Source: CAD feature listing. Evaluate the final solid. Frame: model axes, mm. A direction names the side the tool comes from. Give positions to 0.01 mm unless a question says otherwise; leave off trailing zeros. Loops run counter-clockwise (first coordinate to the right, second up) from the corner with the lowest first, then second, coordinate; pieces in that order, holes last.
```python
from build123d import *

# Parameters (mm, degrees)
F0_R     = 15
F1_DEPTH = 3
F1_TAPER = 15
F2_R     = 1.5
F3_DEPTH = 20
F4_R     = 8
F5_DEPTH = 40
F5_TAPER = 3
F6_R     = 2.5
F7_DEPTH = 5


# Not quite as in the source:
# - a fillet or chamfer that OpenCascade refuses, or shapes differently, is made with other operations: its cross-section is extruded or revolved along the edge and cut away or added


with BuildPart() as f1:
    # F0 (on Top) → F1 (new body)
    with BuildSketch(Plane.XY):
        Circle(F0_R)
    extrude(amount=F1_DEPTH, taper=F1_TAPER)

    # F2 (on face) → F3 (join)
    with BuildSketch(Plane.XY.offset(3)):
        Circle(F2_R)
    extrude(amount=F3_DEPTH)

    # F4 (on face) → F5 (join)
    with BuildSketch(Plane.XY.offset(23)):
        Circle(F4_R)
    extrude(amount=F5_DEPTH, taper=F5_TAPER)

    # F6 (on face) → F7 (cut)
    with BuildSketch(Plane.XY.offset(63)):
        Circle(F6_R)
    extrude(amount=-F7_DEPTH, mode=Mode.SUBTRACT)

    # F8: fillet of radius 7 on 1 edges, made by hand

    # F8_s1 → F8_t2 (revolve, cut)
    with BuildSketch(Plane.XZ):
        with BuildLine():
            ThreePointArc((1.5, 23), (5.9953541002, 25.4536811979), (7.6168139169, 30.3116260276))
            Line((7.6168139169, 30.3116260276), (8, 23))
            Line((8, 23), (1.5, 23))
        make_face()
    revolve(axis=Axis((0, 0, 23), (0, 0, -1)), mode=Mode.SUBTRACT)


solid = f1.part
```
(1) Mould query, pull axis X, two halves, no side actions, for faces 4 (the cylindrical face through (-0.54, -2.44, 60.54)), 5 (the conical face through (-3.086, -13.897, 2.854)), 6 (the flat face through (0, 0, 0)). Classes: pulls with the +X half, pulls with the -X half, needs draft (parallel to the pull), parting line crosses it, or undercut.
A:
face 4: undercut
face 5: parting line crosses it
face 6: needs draft
(2) Section B-B, the plane z = 56.5. Return the cut outline in (x, y), then the cut area to 3 significant figures.
A:
outline: circle Ø12.49 at (0, 0)
area: 122 mm2
(3) First-contact query: pin 1 (1 mm diameter, centred on x = -8, y = 11.5, fed in from -Z); pin 2 (4 mm diameter, centred on x = 0, y = 0, fed in from +Z); pin 3 (1 mm diameter, centred on y = 0, z = 14.5, fed in from +X); pin 4 (1.5 mm diameter, centred on x = -11.5, y = 6.5, fed in from +Z). Flat tips, straight axial feed; report the tip coordinate or a pass-through.
A:
pin 1: stops at z = 0
pin 2: stops at z = 58
pin 3: stops at x = 1.5
pin 4: stops at z = 3
(4) Reachability of faces 1 (the flat face through (0, -3, 63)), 2 (the flat face through (0, 0, 58)), 3 (the cylindrical face through (-1.5, 0.07, 12.86)) from +Z, -Z, +X, -X, +Y, -Y: full face, straight path, thin tool, end or side. Return the list, or none.
A:
face 1: +Z, +X, -X, +Y, -Y
face 2: +Z
face 3: none
(5) Ray query, line 1 along Z through (x, y) = (3, 11); line 2 along Z through (x, y) = (-5.5, 1); line 3 along Y through (x, z) = (0, 61.3). Return the intervals inside material, ascending.
A:
line 1: z = 0 to 3
line 2: z = 0 to 3, 25.01 to 63
line 3: y = -5.99 to -2.5, 2.5 to 5.99
(6) Section A-A, the plane z = 18.5. Return the cut outline in (x, y).
A:
outline: circle Ø3 at (0, 0)
